Geometry: final body of the model. Coordinates: model frame, mm. Round coordinates to 2 decimals unless told otherwise and drop trailing zeros. Loops run counter-clockwise (first coordinate to the right, second up) from the corner with the lowest first, then second, coordinate; pieces in that order, holes last. Notation, with made-up numbers: (51, 8.25) - (102, 8.25) arc R27 ccw to (102, 32.25) - close; hole circle Ø4 at (-19.5, -36). An arc over 180 degrees is marked (long way). Answer as a JSON object with one key per item and string values. Group by question number.
Item 1: Draft query along Z for faces 1 (the face through (88, 3.175, -119)), 2 (the face through (54.65, 1.61, -173.85)). Return one class per face: released by +Z, released by -Z, zero draft, split by the parting line, or undercut.
Item 2: Line query: line 1 (Z direction, x = 125.5, y = 2.1); line 2 (X direction, y = 1.5, z = -123.5) (3 decimals); line 3 (Z direction, x = 42, y = 2.25) (3 decimals). Output: solid intervals per line, ascending.
Item 3: First-contact query: pin 1 (3 mm diameter, centred on x = 120.5, z = -150.5, fed in from -Y); pin 2 (1 mm diameter, centred on y = 1, z = -189.5, fed in from -X) (3 decimals); pin 3 (1.6 mm diameter, centred on x = 130, y = 2, fed in from +Z) (3 decimals); pin 4 (1.6 mm diameter, centred on x = 16, y = 2, fed in from -Z) (3 decimals). Flat tips, straight axial feed; report the tip coordinate or a pass-through.
Item 4: Section A-A (z = -101.5). Return the cut outline in (x, y) (3 decimals), plus the area to 3 significant figures.
Item 5: Section D-D (y = 1.4). Count the separate pieces of the cut face and the enclosed holes in it, plus the area to 3 significant figures.
Item 6: Section C-C (z = -22.5). Return the cut outline in (x, y) (3 decimals), plus the area to 3 significant figures.
Item 7: Section B-B (x = 68.5). Return the cut outline in (y, z) (3 decimals), plus the area to 3 significant figures.
```python
from build123d import *

# Parameters (mm, degrees)
BOSS_EXTRUDE1_DEPTH = 3.175
SKETCH5_W           = 12.7
SKETCH5_H           = 3.175
SKETCH5_W_2         = 25.4
CUT_EXTRUDE4_DEPTH  = 7.62
SKETCH7_W           = 35.56
SKETCH7_H           = 63.5
CUT_EXTRUDE5_DEPTH  = 7.62
CUT_EXTRUDE6_DEPTH  = 7.62
SKETCH9_R           = 2.3495
CUT_EXTRUDE7_DEPTH  = 25.4


with BuildPart() as part:
    # Sketch1 → Boss-Extrude1 (new body)
    with BuildSketch(Plane(origin=(0, 0, 0), x_dir=(1, 0, 0), z_dir=(0, 1, 0))):
        Polygon((3.175, 209.55), (0, 209.55), (0, 196.85), (3.175, 196.85), (3.175, 184.15), (0, 184.15), (0, 171.45), (3.175, 171.45), (3.175, 63.5), (0, 63.5), (0, 50.8), (3.175, 50.8), (3.175, 38.1), (0, 38.1), (0, 25.4), (3.175, 25.4), (3.175, 12.7), (0, 12.7), (0, 0), (177.8, 0), (177.8, 12.7), (174.625, 12.7), (174.625, 25.4), (177.8, 25.4), (177.8, 38.1), (174.625, 38.1), (174.625, 50.8), (177.8, 50.8), (177.8, 63.5), (174.625, 63.5), (174.625, 171.45), (177.8, 171.45), (177.8, 184.15), (174.625, 184.15), (174.625, 196.85), (177.8, 196.85), (177.8, 209.55), (174.625, 209.55), (174.625, 222.25), (177.8, 222.25), (177.8, 234.95), (0, 234.95), (0, 222.25), (3.175, 222.25), align=None)
    extrude(amount=BOSS_EXTRUDE1_DEPTH)

    # Sketch5 → Cut-Extrude4 (cut)
    with BuildSketch(Plane(origin=(0, 3.175, 0), x_dir=(1, 0, 0), z_dir=(0, 1, 0))):
        with Locations((19.05, 1.5875)):
            Rectangle(SKETCH5_W, SKETCH5_H)
        with Locations((44.45, 1.5875)):
            Rectangle(SKETCH5_W, SKETCH5_H)
        with Locations((76.2, 1.5875)):
            Rectangle(SKETCH5_W_2, SKETCH5_H)
        with Locations((101.6, 1.5875)):
            Rectangle(SKETCH5_W_2, SKETCH5_H)
        with Locations((133.35, 1.5875)):
            Rectangle(SKETCH5_W, SKETCH5_H)
        with Locations((158.75, 1.5875)):
            Rectangle(SKETCH5_W, SKETCH5_H)
    cut_extrude4 = extrude(amount=-CUT_EXTRUDE4_DEPTH, mode=Mode.SUBTRACT)

    # Mirror1: Cut-Extrude4 across plane
    add(cut_extrude4.mirror(Plane.XY.offset(-117.475)), mode=Mode.SUBTRACT)

    # Sketch7 → Cut-Extrude5 (cut)
    with BuildSketch(Plane(origin=(0, 3.175, 0), x_dir=(1, 0, 0), z_dir=(0, 1, 0))):
        with Locations((27.305, 117.475)):
            Rectangle(SKETCH7_W, SKETCH7_H)
    extrude(amount=-CUT_EXTRUDE5_DEPTH, mode=Mode.SUBTRACT)

    # Sketch8 → Cut-Extrude6 (cut)
    with BuildSketch(Plane(origin=(0, 3.175, 0), x_dir=(1, 0, 0), z_dir=(0, 1, 0))):
        with BuildLine():
            ThreePointArc((24.859449392, 13.37707256), (25.54760201, 11.715725178), (27.208949392, 11.02757256))
            Line((27.208949392, 11.02757256), (27.208949392, 13.37707256))
            Line((27.208949392, 13.37707256), (24.859449392, 13.37707256))
        make_face()
        with BuildLine():
            ThreePointArc((27.208949392, 15.72657256), (25.54760201, 15.038419942), (24.859449392, 13.37707256))
            Line((24.859449392, 13.37707256), (27.208949392, 13.37707256))
            Line((27.208949392, 13.37707256), (27.208949392, 15.72657256))
        make_face()
        with BuildLine():
            Line((27.208949392, 15.72657256), (27.208949392, 13.37707256))
            Line((27.208949392, 13.37707256), (29.558449392, 13.37707256))
            ThreePointArc((29.558449392, 13.37707256), (28.870296774, 15.038419942), (27.208949392, 15.72657256))
        make_face()
        with BuildLine():
            Line((27.208949392, 13.37707256), (27.208949392, 11.02757256))
            ThreePointArc((27.208949392, 11.02757256), (28.870296774, 11.715725178), (29.558449392, 13.37707256))
            Line((29.558449392, 13.37707256), (27.208949392, 13.37707256))
        make_face()
        with BuildLine():
            ThreePointArc((29.558449392, 74.849360588), (25.54760201, 76.51070797), (27.208949392, 72.499860588))
            Line((27.208949392, 72.499860588), (27.208949392, 74.849360588))
            Line((27.208949392, 74.849360588), (29.558449392, 74.849360588))
        make_face()
        with BuildLine():
            Line((27.208949392, 74.849360588), (27.208949392, 72.499860588))
            ThreePointArc((27.208949392, 72.499860588), (28.870296774, 73.188013206), (29.558449392, 74.849360588))
            Line((29.558449392, 74.849360588), (27.208949392, 74.849360588))
        make_face()
        with BuildLine():
            ThreePointArc((148.241550608, 74.849360588), (148.929703226, 73.188013206), (150.591050608, 72.499860588))
            Line((150.591050608, 72.499860588), (150.591050608, 74.849360588))
            Line((150.591050608, 74.849360588), (148.241550608, 74.849360588))
        make_face()
        with BuildLine():
            Line((150.591050608, 74.849360588), (150.591050608, 72.499860588))
            ThreePointArc((150.591050608, 72.499860588), (152.25239799, 73.188013206), (152.940550608, 74.849360588))
            ThreePointArc((152.940550608, 74.849360588), (150.591050608, 77.198860588), (148.241550608, 74.849360588))
            Line((148.241550608, 74.849360588), (150.591050608, 74.849360588))
        make_face()
        with BuildLine():
            ThreePointArc((150.591050608, 15.72657256), (148.929703226, 15.038419942), (148.241550608, 13.37707256))
            Line((148.241550608, 13.37707256), (150.591050608, 13.37707256))
            Line((150.591050608, 13.37707256), (150.591050608, 15.72657256))
        make_face()
        with BuildLine():
            Line((150.591050608, 13.37707256), (148.241550608, 13.37707256))
            ThreePointArc((148.241550608, 13.37707256), (150.591050608, 11.02757256), (152.940550608, 13.37707256))
            ThreePointArc((152.940550608, 13.37707256), (152.25239799, 15.038419942), (150.591050608, 15.72657256))
            Line((150.591050608, 15.72657256), (150.591050608, 13.37707256))
        make_face()
    extrude(amount=-CUT_EXTRUDE6_DEPTH, mode=Mode.SUBTRACT)

    # Sketch9 → Cut-Extrude7 (cut)
    with BuildSketch(Plane(origin=(0, 3.175, 0), x_dir=(1, 0, 0), z_dir=(0, 1, 0))):
        with Locations(Location((52.32122124, 210.560282968, 0), (0, 0, 270))):
            Circle(SKETCH9_R)
        with Locations(Location((52.32122124, 173.54571463, 0), (0, 0, 270))):
            Circle(SKETCH9_R)
        with Locations(Location((125.47877876, 173.54571463, 0), (0, 0, 270))):
            Circle(SKETCH9_R)
        with Locations(Location((125.47877876, 210.560282968, 0), (0, 0, 270))):
            Circle(SKETCH9_R)
    extrude(amount=-CUT_EXTRUDE7_DEPTH, mode=Mode.SUBTRACT)


solid = part.part
```
Values:
{
 "1": {"face 1": "zero draft", "face 2": "undercut"},
 "2": {"line 1": "z = -234.95 to -212.91, -208.21 to -175.9, -171.2 to 0", "line 2": "x = 3.175 to 9.525, 45.085 to 174.625", "line 3": "z = -231.775 to -149.225, -85.725 to -3.175"},
 "3": {"pin 1": "stops at y = 0", "pin 2": "stops at x = 3.175", "pin 3": "stops at z = -3.175", "pin 4": "stops at z = -231.775"},
 "4": {"outline": "(3.175, 0) - (9.525, 0) - (9.525, 3.175) - (3.175, 3.175) - close; (45.085, 0) - (174.625, 0) - (174.625, 3.175) - (45.085, 3.175) - close", "area": "431 mm^2"},
 "5": {"separate pieces": "1", "enclosed holes": "9", "area": "37,700 mm^2"},
 "6": {"outline": "(3.175, 0) - (174.625, 0) - (174.625, 3.175) - (3.175, 3.175) - close", "area": "544 mm^2"},
 "7": {"outline": "(0, -231.775) - (3.175, -231.775) - (3.175, -3.175) - (0, -3.175) - close", "area": "726 mm^2"}
}
